from build123d import *

# Parameters (mm, degrees)
SKETCH3_W               = 3
SKETCH3_H               = 22
CUT_EXTRUDE1_DEPTH      = 35.365680555
CUT_EXTRUDE1_DEPTH_BACK = 35.365680555
SKETCH1_R               = 1
SKETCH1_R_2             = 2.9


with BuildPart() as part:
    # Sweep1: sweep along a path in Sketch2
    with BuildLine(Plane(origin=(0, 0, 0), x_dir=(1, 0, 0), z_dir=(0, 1, 0))) as sweep1_path:
        Line((11, -21), (0, -21))
        Line((0, -21), (-19, -21))
        Line((-19, -21), (-19, 21))
        Line((-19, 21), (0, 21))
        Line((0, 21), (11, 21))
    # Sketch3 → Sweep1 (sweep)
    with BuildSketch(Plane(origin=(0, 0, 0), x_dir=(0, 0, -1), z_dir=(1, 0, 0))):
        with Locations((22.5, 0)):
            Rectangle(SKETCH3_W, SKETCH3_H)
    sweep(path=sweep1_path.line, transition=Transition.RIGHT)

    # Sketch1 → Cut-Extrude1 (cut, two sides: drawn at the far end of the back side and taken through both)
    with BuildSketch(Plane.XY.offset(-CUT_EXTRUDE1_DEPTH_BACK)):
        with BuildLine():
            Line((11, 11), (0, 11))
            ThreePointArc((0, 11), (7.778174593, 7.778174593), (11, 0))
            Line((11, 0), (11, 11))
        make_face()
        with Locations((8, 0)):
            Circle(SKETCH1_R)
        with Locations(Location((0, -8, 0), (0, 0, 270))):
            Circle(SKETCH1_R)
        with Locations(Location((0, 0, 0), (0, 0, 270))):
            Circle(SKETCH1_R_2)
        with BuildLine():
            Line((11, -11), (11, 0))
            ThreePointArc((11, 0), (7.778174593, -7.778174593), (0, -11))
            Line((0, -11), (11, -11))
        make_face()
        with Locations(Location((0, 8, 0), (0, 0, 270))):
            Circle(SKETCH1_R)
        with Locations((-8, 0)):
            Circle(SKETCH1_R)
    extrude(amount=CUT_EXTRUDE1_DEPTH + CUT_EXTRUDE1_DEPTH_BACK, mode=Mode.SUBTRACT)


solid = part.part
The model under review builds one solid part; all positions refer to its coordinate system, in mm. A direction names the side the tool comes from. Coordinates: 2 decimals unless noted, no trailing zeros. Loops run counter-clockwise (first coordinate to the right, second up) from the corner with the lowest first, then second, coordinate; pieces in that order, holes last. Notation, with made-up numbers: (-6, -6.75) -> (18, -6.75) arc R15 ccw to (18, 16.25) -> close; hole circle Ø11 at (79, 73). An arc over 180 degrees is marked (long way). Use a Markdown table: item, result. Add a question column.
1. Machinability: for faces 1 (the face through (-4, 0, -21)), 2 (the face through (-22, 0, 0)), which of the approach directions +Z, -Z, +X, -X, +Y, -Y give a long, thin tool a straight path to every point of the face, cutting with its end or side? Answer none if there is none.
2. Add section B-B on y = -7.5. Write out the cut boundary in (x, z), plus the area to 3 significant figures.
3. Draft analysis for pull direction Y (two halves, no side actions). For faces 3 (the face through (-1, -8, -23)), 4 (the face through (-19.2, 11, 0.1)), 5 (the face through (-1, -8, 22)), 6 (the face through (-6, 0, 24)), state which applies: pulls with the +Y half, pulls with the -Y half, needs draft (parallel to the pull), parting line crosses it, or undercut.
4. To check wall thickness, follow line 1 (Y direction, x = 0, z = 22.15); line 2 (X direction, y = 0, z = 22.4); line 3 (Z direction, x = -4, y = 9). State the ranges of each line that lie inside material, in increasing order.
5. Add section A-A on x = -8. Write out the cut boundary in (y, z).
6. Add section C-C on x = 5. Write out the cut boundary in (y, z).
7. Add section D-D on z = 7.5. Write out the cut boundary in (x, y), plus the area to 3 significant figures.
8. Clearance check with flat-ended pins moving along their axes: pin 1 Ø1.6 at (x, y) = (8, 0) entering from +Z; pin 2 Ø11 at (y, z) = (-2, 0) entering from +X. State where each tip first meets the part, or that it passes through.
Returned:
| question | item | result |
|---|---|---|
| 1 | face 1 | +X, +Y, -Y |
| 1 | face 2 | +Z, -Z, -X, +Y, -Y |
| 2 | outline | (-22, -24) -> (-0.87, -24) -> (-0.87, -21) -> (-19, -21) -> (-19, 21) -> (-0.87, 21) -> (-0.87, 24) -> (-22, 24) -> close; (0.87, -24) -> (8.05, -24) -> (8.05, -21) -> (0.87, -21) -> close; (0.87, 21) -> (8.05, 21) -> (8.05, 24) -> (0.87, 24) -> close |
| 2 | area | 296 mm² |
| 3 | face 3 | undercut |
| 3 | face 4 | pulls with the +Y half |
| 3 | face 5 | undercut |
| 3 | face 6 | needs draft |
| 4 | line 1 | y = -11 to -9, -7 to -2.9, 2.9 to 7, 9 to 11 |
| 4 | line 2 | x = -22 to -9, -7 to -2.9, 2.9 to 7, 9 to 11 |
| 4 | line 3 | z = -24 to -21, 21 to 24 |
| 5 | outline | (-11, -24) -> (-1, -24) -> (-1, -21) -> (-11, -21) -> close; (-11, 21) -> (-1, 21) -> (-1, 24) -> (-11, 24) -> close; (1, -24) -> (11, -24) -> (11, -21) -> (1, -21) -> close; (1, 21) -> (11, 21) -> (11, 24) -> (1, 24) -> close |
| 6 | outline | (-9.8, -24) -> (9.8, -24) -> (9.8, -21) -> (-9.8, -21) -> close; (-9.8, 21) -> (9.8, 21) -> (9.8, 24) -> (-9.8, 24) -> close |
| 7 | outline | (-22, -11) -> (-19, -11) -> (-19, 11) -> (-22, 11) -> close |
| 7 | area | 66.0 mm² |
| 8 | pin 1 | passes through |
| 8 | pin 2 | stops at x = -19 |
